For this review, take the finished solid that the model builds, in its own axes (mm). A direction names the side the tool comes from. Round coordinates to 2 decimals unless told otherwise and drop trailing zeros. Order: outer loops, then holes, each group sorted by start corner. A loop starts at its lowest first (then second) coordinate and runs counter-clockwise, first axis right, second up. Notation, with made-up numbers: M 34.25,13 L 65.25,13 A15 ccw 65.25,38 Z; hole C -33.5,17 d2. An arc over 180 degrees is marked long. Answer in a Markdown table with one row per item. Add a question column.
```python
from build123d import *

# Parameters (mm, degrees)
F1_DEPTH = 150
F2_R     = 5
F3_R     = 14.9999953218
F3_R_2   = 15
F4_DEPTH = 25
F5_R     = 27.0158280376
F6_DEPTH = 25


with BuildPart() as f1:
    # F0 (on Front) → F1 (new body)
    with BuildSketch(Plane.XZ):
        Polygon((93.6258085565, 97.991302244), (-98.2046941788, -62.3241936394), (-87.4790228189, -75.1583299641), (104.3514799163, 85.1571659193), align=None)
        with BuildLine():
            Line((-87.4790228189, -75.1583299641), (-98.2046941788, -62.3241936394))
            ThreePointArc((-98.2046941788, -62.3241936394), (-109.0167692981, -116.9894962958), (-57.8507907344, -139.0629853841))
            Line((-57.8507907344, -139.0629853841), (-58.3305805922, -120.1455667615))
            ThreePointArc((-58.3305805922, -120.1455667615), (-92.8244846189, -110.5584473591), (-87.4790228189, -75.1583299641))
        make_face()
        Polygon((-58.3305805922, -120.1455667615), (-57.8507907344, -139.0629853841), (441.5086849726, -126.3980644136), (441.5086849726, -107.4684772011), align=None)
    extrude(amount=F1_DEPTH)

    # F2
    f2_edges = [f1.edges().sort_by_distance(p)[0] for p in [
        (98.988644, -150, 91.574234),
        (98.988644, 0, 91.574234),
        (441.508685, -150, -116.933271),
        (441.508685, 0, -116.933271),
    ]]
    fillet(f2_edges, radius=F2_R)

    # F3 (on face) → F4 (cut)
    with BuildSketch(Plane(origin=(-9.7165371294, 0, 11.6266253123), x_dir=(0.7673220109, 0, 0.6412619835), z_dir=(-0.6412619835, 0, 0.7673220109))):
        with Locations((57.3368984643, -106.4837826855)):
            Circle(F3_R)
        with Locations((66.128025143, -25.343221313)):
            Circle(F3_R_2)
    extrude(amount=-F4_DEPTH, mode=Mode.SUBTRACT)

    # F5 (on face) → F6 (cut)
    with BuildSketch(Plane(origin=(3.0077160605, 0, -118.5898844978), x_dir=(0.9996785311, 0, 0.0253541791), z_dir=(-0.0253541791, 0, 0.9996785311))):
        with Locations((63.3628219366, -70.44968009)):
            Circle(F5_R)
        with BuildLine():
            Line((290.8473328755, -60.3176639156), (233.4038116923, -59.7659925333))
            ThreePointArc((233.4038116923, -59.7659925333), (220.5742240017, -72.4120867419), (233.2817761647, -85.180803869))
            Line((233.2817761647, -85.180803869), (233.5255773105, -85.1784649534))
            Line((233.5255773105, -85.1784649534), (290.8472091458, -84.6285476904))
            ThreePointArc((290.8472091458, -84.6285476904), (302.8865972816, -72.4731670769), (290.8473328755, -60.3176639156))
        make_face()
        with BuildLine():
            Line((233.5255773105, -85.1784649534), (233.2817761647, -85.180803869))
            ThreePointArc((233.2817761647, -85.180803869), (233.4036823471, -85.1802191266), (233.5255773105, -85.1784649534))
        make_face()
    extrude(amount=-F6_DEPTH, mode=Mode.SUBTRACT)


solid = f1.part
```
1. The part is to be moulded in two halves that separate along Z. For faces 1 (the cylindrical face through (-92.52, -73.95, -111.02)), 2 (the flat face through (441.509, -74, -117)), 3 (the cylindrical face through (97.82, -1.504, 90.75)), say which applies: pulls with the +Z half, pulls with the -Z half, needs draft (parallel to the pull), parting line crosses it, or undercut.
2. Consider section A-A on x = 265. Write out the cut boundary in (y, z), plus the area to 3 significant figures.
3. Clearance check with flat-ended pins moving along their axes: pin 1 Ø6 at (y, z) = (-120.5, -95.5) entering from +X; pin 2 Ø12 at (y, z) = (-70.5, 46.5) entering from +X; pin 3 Ø10 at (x, y) = (343.5, -25) entering from +Z. State where each tip first meets the part, or that it passes through.
4. For faces 4 (the flat face through (99.064, -74.02, 91.484)), 5 (the flat face through (7.093, -73.95, 3.877)), 6 (the cylindrical face through (43.818, -39.987, 45.62)), list the 3-axis set-ups (+Z, -Z, +X, -X, +Y, -Y) from which the entire face can be reached by the end or side of a thin tool; tool diameter is ignored.
5. Consider section C-C on x = -9.5. Write out the cut boundary in (y, z), plus the area to 3 significant figures.
6. Consider section B-B on y = -131.5. Write out the cut boundary in (x, z), plus the area to 3 significant figures.
7. Consider section D-D on z = -100.5. Write out the cut boundary in (x, y).
8. To check wall thickness, follow probe 1 along Z at (x, y) = (388.5, -56); probe 2 along X at (y, z) = (-40, 63); probe 3 along Z at (x, y) = (177.5, -140). State the ranges of each line that lie inside material, in increasing order. Write a range as [from, to].
Solved:
| question | item | result |
|---|---|---|
| 1 | face 1 | undercut |
| 1 | face 2 | needs draft |
| 1 | face 3 | pulls with the +Z half |
| 2 | outline | M -150,-130.87 L -84.91,-130.87 L -84.9,-111.95 L -150,-111.95 Z; M -60.04,-130.87 L 0,-130.87 L 0,-111.95 L -60.04,-111.95 Z |
| 2 | area | 2,370 mm^2 |
| 3 | pin 1 | stops at x = -96.95 |
| 3 | pin 2 | stops at x = 65.27 |
| 3 | pin 3 | stops at z = -109.83 |
| 4 | face 4 | +Z, +X, +Y, -Y |
| 4 | face 5 | +X, +Y, -Y |
| 4 | face 6 | none |
| 5 | outline | M -150,-137.84 L 0,-137.84 L 0,-118.91 L -150,-118.91 Z; M -150,-9.99 L 0,-9.99 L 0,11.81 L -150,11.81 Z |
| 5 | area | 6,110 mm^2 |
| 6 | outline | M -98.2,-62.32 A44.34 ccw -57.85,-139.06 L 441.51,-126.4 L 441.51,-107.47 L -58.33,-120.15 A27 cw -87.48,-75.16 L 104.35,85.16 L 93.63,97.99 Z |
| 6 | area | 15,400 mm^2 |
| 7 | outline | M -113.92,-150 L -96.77,-150 L -96.77,0 L -113.92,0 Z |
| 8 | probe 1 | z = [-127.74, -108.81] |
| 8 | probe 2 | x = [51.76, 77.84] |
| 8 | probe 3 | z = [-133.09, -114.16] |
